Autodesk Inventor part; units mm, degrees
ref_plane "YZ Plane" through (0, 0, 0) normal (1, 0, 0) x (0, 1, 0)
ref_plane "XZ Plane" through (0, 0, 0) normal (0, 1, 0) x (-1, 0, 0)
ref_plane "XY Plane" through (0, 0, 0) normal (0, 0, 1) x (1, 0, 0)
sketch "Sketch2" plane through (0, 0, 0) normal (0, 1, 0) x (-1, 0, 0)
  line L0 (-44.45, 50.8) -> (44.45, 50.8)
  line L1 (44.45, 50.8) -> (44.45, -50.8)
  line L2 (44.45, -50.8) -> (-44.45, -50.8)
  line L3 (-44.45, -50.8) -> (-44.45, 50.8)
  point P0 (0, 0)
  dimension "d0" = 44.45
  dimension "d1" = 44.45
  dimension "d2" = 50.8
  dimension "d3" = 50.8
extrude "Extrusion1" add sketch "Sketch2" along normal blind 3.175
fillet "Fillet1" radius 12.7 4 edges at (44.45, 1.5875, 50.8) (-44.45, 1.5875, 50.8) (44.45, 1.5875, -50.8) (-44.45, 1.5875, -50.8)
sketch "Sketch3" plane through (0, 3.175, 0) normal (0, 1, 0) x (1, 0, 0)
  line L0 (-44.45, -38.1) -> (-44.45, 38.1)
  line L1 (31.75, -50.8) -> (-31.75, -50.8)
  line L2 (44.45, 38.1) -> (44.45, -38.1)
  line L3 (-31.75, 50.8) -> (31.75, 50.8)
  point P0 (0, 0)
  point P1 (0, 0)
  point P2 (-19.05, 38.1)
  point P3 (19.05, 38.1)
  point P4 (19.05, -38.1)
  point P5 (-19.05, -38.1)
  dimension "d7" = 12.7
  dimension "d8" = 25.4
  dimension "d9" = 25.4
  dimension "d10" = 12.7
hole "Hole1" at (0, 3.175, 0) at (-19.05, 3.175, -38.1) at (19.05, 3.175, -38.1) at (19.05, 3.175, 38.1) at (-19.05, 3.175, 38.1) direction (0, -1, 0) diameter 6.35 end through all
sketch "Sketch4" plane through (0, 0, 0) normal (0, 0, 1) x (1, 0, 0)
  line L0 (22.225, 3.175) -> (22.225, 22.225)
  line L1 (22.225, 22.225) -> (15.875, 22.225)
  line L2 (15.875, 22.225) -> (15.875, 19.05)
  line L3 (15.875, 19.05) -> (19.05, 19.05)
  line L4 (19.05, 19.05) -> (19.05, 15.875)
  line L5 (19.05, 15.875) -> (15.875, 15.875)
  line L6 (15.875, 15.875) -> (15.875, 12.7)
  line L7 (15.875, 12.7) -> (19.05, 12.7)
  line L8 (19.05, 12.7) -> (19.05, 3.175)
  line L9 (19.05, 3.175) -> (22.225, 3.175)
  line L10 (0, -4.445) -> (0, 26.67)
  point P0 (0, 0)
  dimension "d18" = 19.05
  dimension "d19" = 22.225
  dimension "d20" = 3.175
  dimension "d21" = 6.35
  dimension "d22" = 3.175
  dimension "d23" = 3.175
  dimension "d24" = 3.175
  dimension "d25" = 3.175
  dimension "d26" = 3.175
  dimension "d27" = 3.175
  dimension "d28" = 9.525
revolve "Revolution1" add sketch "Sketch4" angle 360 about axis through (0, -10, 0) along (0, 1, 0)
equation "\"d4\" = metalThickness"
equation "\"metalThickness\" = 3.175"
properties part number "Rotation Top"
Could you check a few things on this model? Use its own coordinates, in mm. A direction names the side the tool comes from. Give positions to 0.01 mm unless a question says otherwise; leave off trailing zeros. Write each loop counter-clockwise with the first axis right and the second up, starting at its lowest first coordinate (ties: lowest second). Pieces come first, ordered by that corner, then holes. Notation, with made-up numbers: (77.5, 7) - (83.5, 7) arc R14 ccw to (83.5, 14) - close; hole circle Ø5 at (-15, 69). An arc over 180 degrees is marked (long way). One line per item, written item: value. Start each with the question number.
Item 1: Imagine slicing it at C-C, the plane x = 9. List the corners of the cut face in (y, z) for me (3 decimals).
Item 2: Imagine slicing it at A-A, the plane z = 0. List the corners of the cut face in (x, y) for me (3 decimals).
Item 3: Imagine slicing it at B-B, the plane y = 5.25. List the corners of the cut face in (x, z) for me (3 decimals), and give its area (3 significant figures).
Item 4: Please list where these lines run through material, in increasing order: line 1 (X direction, y = 0.8, z = -38.1) (3 decimals); line 2 (Y direction, x = -11, z = 15.5) (3 decimals); line 3 (Z direction, x = 19.05, y = 1.4) (3 decimals). Write a range as from..to.
Item 5: I'm going to push flat-ended pins straight in: pin 1 (5.5 mm diameter, centred on x = 0, z = 0, fed in from -Y); pin 2 (12 mm diameter, centred on x = -32.5, z = -3, fed in from -Y); pin 3 (6 mm diameter, centred on x = -11.5, z = 25, fed in from +Y) (3 decimals); pin 4 (6 mm diameter, centred on y = 7, z = -9, fed in from +X). Where does each tip first touch, or does it pass through?
Item 6: If we mould it in two halves opening along Z, with no side actions, what happens to faces 4 (the face through (21.199, 12.833, -6.676)), 5 (the face through (-15.95, 1.57, -38.79)), 6 (the face through (40.83, 1.61, -46.98))? For each: +Z half, -Z half, draft (parallel to the pull), parting line (faces both ways), or undercut.
Item 7: Which directions (+Z, -Z, +X, -X, +Y, -Y) give clear straight access to the entire face, cutting with the end or side of a thin tool? Please do faces 1 (the face through (-4, 19.05, -16)), 2 (the face through (1, 3.175, 23)), 3 (the face through (-44.45, 2, 1)).
Item 8: Imagine slicing it at D-D, the plane z = 31.5. List the corners of the cut face in (x, y) for me (3 decimals), and give its area (3 significant figures).
Geometry says:
1. outline: (0, -50.8) - (3.175, -50.8) - (3.175, -20.321) - (22.225, -20.321) - (22.225, -13.077) - (19.05, -13.077) - (19.05, -16.79) - (15.875, -16.79) - (15.875, -13.077) - (12.7, -13.077) - (12.7, -16.79) - (3.175, -16.79) - (3.175, 16.79) - (12.7, 16.79) - (12.7, 13.077) - (15.875, 13.077) - (15.875, 16.79) - (19.05, 16.79) - (19.05, 13.077) - (22.225, 13.077) - (22.225, 20.321) - (3.175, 20.321) - (3.175, 50.8) - (0, 50.8) - close
2. outline: (-44.45, 0) - (-3.175, 0) - (-3.175, 3.175) - (-19.05, 3.175) - (-19.05, 12.7) - (-15.875, 12.7) - (-15.875, 15.875) - (-19.05, 15.875) - (-19.05, 19.05) - (-15.875, 19.05) - (-15.875, 22.225) - (-22.225, 22.225) - (-22.225, 3.175) - (-44.45, 3.175) - close; (3.175, 0) - (44.45, 0) - (44.45, 3.175) - (22.225, 3.175) - (22.225, 22.225) - (15.875, 22.225) - (15.875, 19.05) - (19.05, 19.05) - (19.05, 15.875) - (15.875, 15.875) - (15.875, 12.7) - (19.05, 12.7) - (19.05, 3.175) - (3.175, 3.175) - close
3. outline: circle Ø44.45 at (0, 0); hole circle Ø38.1 at (0, 0)
3. area: 412 mm^2
4. line 1: -44.45..-22.225, -15.875..15.875, 22.225..44.45
4. line 2: 0..3.175, 12.7..15.875, 19.05..22.225
4. line 3: -50.8..-41.275, -34.925..34.925, 41.275..50.8
5. pin 1: through
5. pin 2: y = 0
5. pin 3: y = 3.175
5. pin 4: x = 21.4
6. face 4: parting line
6. face 5: undercut
6. face 6: -Z half
7. face 1: none
7. face 2: +Y
7. face 3: +Z, -Z, -X, +Y, -Y
8. outline: (-44.45, 0) - (44.45, 0) - (44.45, 3.175) - (-44.45, 3.175) - close
8. area: 282 mm^2
